Input: part model. Units: mm. Frame: model coordinates. Coordinates: 2 decimals unless noted, no trailing zeros. Order: outer loops, then holes, each group sorted by start corner. A loop starts at its lowest first (then second) coordinate and runs counter-clockwise, first axis right, second up. Notation, with made-up numbers: (63, 6) -> (76, 6) arc R19 cw to (76, 22) -> close; hole circle Ø3 at (-12, 73). An arc over 180 degrees is marked (long way). Write each question's results on one line, items separated by ' | '.
```python
from build123d import *

# Parameters (mm, degrees)
ESQUISSE1_R        = 1.5
BOSS_EXTRU_1_DEPTH = 46
ESQUISSE2_R        = 3
BOSS_EXTRU_2_DEPTH = 1
CONG_1_R           = 1
CONG_2_R           = 0.25


with BuildPart() as part:
    # Esquisse1 → Boss.-Extru.1 (new body)
    with BuildSketch(Plane.XY):
        with Locations((-28.068256791, 21.884700983)):
            Circle(ESQUISSE1_R)
    extrude(amount=BOSS_EXTRU_1_DEPTH)

    # Esquisse2 → Boss.-Extru.2 (add)
    with BuildSketch(Plane.XY.offset(46)):
        with Locations((-28.068256791, 21.884700983)):
            Circle(ESQUISSE2_R)
    extrude(amount=BOSS_EXTRU_2_DEPTH)

    # Congé1
    cong_1_edges = [part.edges().sort_by_distance(p)[0] for p in [
        (-31.068256791, 21.884700983, 47),
    ]]
    fillet(cong_1_edges, radius=CONG_1_R - 0.0001)  # a hair under: the kernel refuses the full size

    # Congé2
    cong_2_edges = [part.edges().sort_by_distance(p)[0] for p in [
        (-29.568256791, 21.884700983, 0),
    ]]
    fillet(cong_2_edges, radius=CONG_2_R)


solid = part.part
```
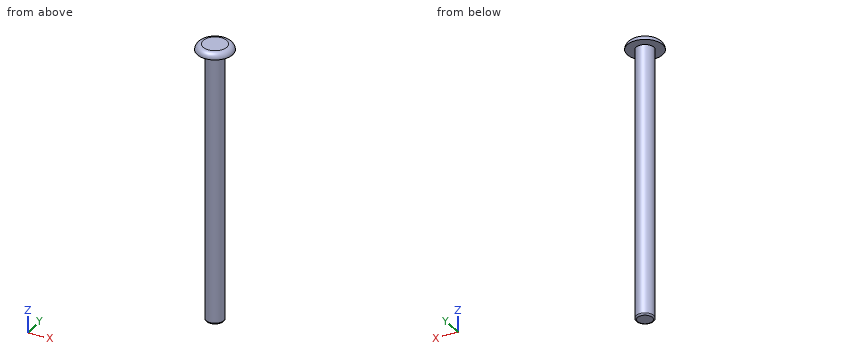
(1) Line query: line 1 along X through (y, z) = (22, 22.5); line 2 along Z through (x, y) = (-29.85, 23); line 3 along Y through (x, z) = (-28.1, 4). Output: solid intervals per line, ascending. Write a range as from..to.
Return value:
line 1: -29.56..-26.57 | line 2: 46..46.99 | line 3: 20.39..23.38
(2) Pin query (flat end, axial travel): P1, Ø2, axis at x = -27.5, y = 21, coming from the -Z side; P2, Ø1, axis at x = -27, y = 24, coming from the -Z side. Return the tip coordinate at first contact, or that it passes through.
Return value:
P1: z = 0 | P2: z = 46
(3) Cut plane A-A, the plane z = 7.5. Return loops of the section in (x, y).
Return value:
outline: circle Ø3 at (-28.07, 21.88)
